Model file for the job. Use its own axes, mm. Face numbers are marked on the shaded views. Round coordinates to 2 decimals unless told otherwise and drop trailing zeros. Loops run counter-clockwise (first coordinate to the right, second up) from the corner with the lowest first, then second, coordinate; pieces in that order, holes last. Notation, with made-up numbers: (88, -20) - (106, -20) arc R5 cw to (106, -16) - close; hole circle Ø3 at (7, 41). An arc over 180 degrees is marked (long way). Use one line per item in the form item = value.
from build123d import *

# Parameters (mm, degrees)
SKETCH1_W            = 34.925
SKETCH1_H            = 15.08125
EXTRUDE1_DEPTH       = 10.7696
M4_CLEARANCE_HOLE1_D = 4.5
FILLET1_R            = 7.540625


with BuildPart() as part:
    # Sketch1 → Extrude1 (new body)
    with BuildSketch(Plane(origin=(0, 0, 0), x_dir=(1, 0, 0), z_dir=(0, 1, 0))):
        Rectangle(SKETCH1_W, SKETCH1_H)
    extrude(amount=EXTRUDE1_DEPTH)

    # M4 Clearance Hole1 (through all)
    with Locations(Plane(origin=(0, 10.7696, 0), x_dir=(-1, 0, 0), z_dir=(0, 1, 0))):
        with Locations((12.7, 0), (-12.7, 0)):
            Hole(M4_CLEARANCE_HOLE1_D / 2)

    # Fillet1
    fillet1_edges = [part.edges().sort_by_distance(p)[0] for p in [
        (17.4625, 5.3848, 7.540625),
        (17.4625, 5.3848, -7.540625),
        (-17.4625, 5.3848, -7.540625),
        (-17.4625, 5.3848, 7.540625),
    ]]
    fillet(fillet1_edges, radius=FILLET1_R - 0.0001)  # a hair under: the kernel refuses the full size


solid = part.part
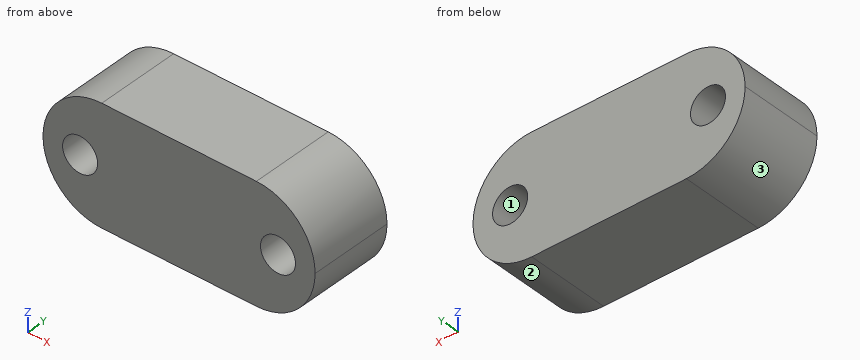
1. Pull direction X, two halves, no side cores. Call the marked faces 1, 2 and 3: +X half, -X half, draft (parallel to the pull), parting line (faces both ways), or undercut.
Geometry check:
face_1 = undercut
face_2 = +X half
face_3 = -X half
2. Flat gauge pins, fed straight in: pin 1 (1 mm diameter, centred on x = -2.5, z = -1, fed in from -Y); pin 2 (2 mm diameter, centred on y = 3, z = -1.5, fed in from +X); pin 3 (1 mm diameter, centred on x = 11, y = 7, fed in from -Z); pin 4 (1 mm diameter, centred on y = 8.5, z = -4.5, fed in from -X). Where does each tip first touch, or does it go through?
Geometry check:
pin_1 = 0
pin_2 = 17.45
pin_3 = -7.52
pin_4 = -16.31
3. Wall check: probe 1 along X at (y, z) = (1, -1.75); probe 2 along X at (y, z) = (6.5, 1); probe 3 along Z at (x, y) = (-12.7, 5.25). Give the ranges that are in metal, low to high.
Geometry check:
probe_1 = -17.26 to -14.11, -11.29 to 11.29, 14.11 to 17.26
probe_2 = -17.4 to -14.72, -10.68 to 10.68, 14.72 to 17.4
probe_3 = -7.01 to -2.25, 2.25 to 7.01
4. Cut at D-D, the plane z = 4.75. Give the cut face in (x, y), plus the area to 3 significant figures.
Geometry check:
outline = (-15.78, 0) - (15.78, 0) - (15.78, 10.77) - (-15.78, 10.77) - close
area = 340 mm^2
5. Cut at A-A, the plane y = 2.5. Give the number of separate pieces and of enclosed holes in the cut face, plus the area to 3 significant figures.
Geometry check:
separate_pieces = 1
enclosed_holes = 2
area = 446 mm^2
6. Cut at C-C, the plane z = 1. Give the cut face in (x, y), plus the area to 3 significant figures.
Geometry check:
outline = (-17.4, 0) - (-14.72, 0) - (-14.72, 10.77) - (-17.4, 10.77) - close; (-10.68, 0) - (10.68, 0) - (10.68, 10.77) - (-10.68, 10.77) - close; (14.72, 0) - (17.4, 0) - (17.4, 10.77) - (14.72, 10.77) - close
area = 288 mm^2
7. Cut at B-B, the plane x = -12.7. Give the cut face in (y, z), plus the area to 3 significant figures.
Geometry check:
outline = (0, -7.01) - (10.77, -7.01) - (10.77, -2.25) - (0, -2.25) - close; (0, 2.25) - (10.77, 2.25) - (10.77, 7.01) - (0, 7.01) - close
area = 103 mm^2
